from build123d import *

# Parameters (mm, degrees)
F0_W     = 118
F0_H     = 27.3
F0_W_2   = 114
F0_H_2   = 23.3
F1_DEPTH = 40
F2_W     = 4.2
F2_H     = 8.5
F3_DEPTH = 40
F4_W     = 27
F4_H     = 7.8
F5_DEPTH = 15
F6_W     = 118
F6_H     = 27.3
F7_DEPTH = 2


with BuildPart() as f1:
    # F0 (on Top) → F1 (new body)
    with BuildSketch(Plane.XY):
        with Locations((-1.233262, 0)):
            Rectangle(F0_W, F0_H)
        with Locations((-1.233262, 0)):
            Rectangle(F0_W_2, F0_H_2, mode=Mode.SUBTRACT)
    extrude(amount=F1_DEPTH)

    # F2 (on Top) → F3 (join)
    with BuildSketch(Plane.XY):
        with Locations((46.666738, 7.4)):
            Rectangle(F2_W, F2_H)
    extrude(amount=F3_DEPTH)

    # F4 (on Top) → F5 (join)
    with BuildSketch(Plane.XY):
        with Locations((35.266738, -7.75)):
            Rectangle(F4_W, F4_H)
    extrude(amount=F5_DEPTH)

    # F6 (on Top) → F7 (join)
    with BuildSketch(Plane.XY):
        with Locations((-1.233262, 0)):
            Rectangle(F6_W, F6_H)
    extrude(amount=-F7_DEPTH)


solid = f1.part
Read the model definition and answer for the solid it produces. Units are mm, in the model's axes. A direction names the side the tool comes from. Give positions to 0.01 mm unless a question says otherwise; leave off trailing zeros. Write each loop counter-clockwise with the first axis right and the second up, starting at its lowest first coordinate (ties: lowest second). Pieces come first, ordered by that corner, then holes. Notation, with made-up numbers: (-7, 46.5) - (48, 46.5) arc R23 ccw to (48, 68.5) - close; hole circle Ø6 at (50.5, 35). An arc over 180 degrees is marked (long way). Return JSON: item names as keys, results as strings.
Q1. Given P1, Ø8.5, axis at x = 38, y = -6, coming from the +Z side; P2, Ø1.5, axis at x = 43, y = 8, coming from the +Z side, each flat-ended and moving along its own axis, determine where each tip first touches the part or whether it passes through.
Reply:
{"P1": "z = 15", "P2": "z = 0"}
Q2. A cutting plane is placed at D-D, the plane x = 31. Determine the outline of the cut face in (y, z), and give its area (3 significant figures).
Reply:
{"outline": "(-13.65, -2) - (13.65, -2) - (13.65, 40) - (11.65, 40) - (11.65, 0) - (-3.85, 0) - (-3.85, 15) - (-11.65, 15) - (-11.65, 40) - (-13.65, 40) - close", "area": "332 mm²"}
Q3. For faces 4 (the face through (-8, 11.65, 20)), 5 (the face through (-2, 13.65, 19)), determine the directions among +Z, -Z, +X, -X, +Y, -Y from which every point of the face is accessible in a straight line to the end or side of a thin tool.
Reply:
{"face 4": "+Z", "face 5": "+Z, -Z, +X, -X, +Y"}
Q4. Consider line 1 along X through (y, z) = (-7, 9.5); line 2 along X through (y, z) = (4.75, 38); line 3 along Y through (x, z) = (31, 13). Determine where each line is inside the solid, lowest interval first. Write a range as [from, to].
Reply:
{"line 1": "[-60.23, -58.23], [21.77, 48.77], [55.77, 57.77]", "line 2": "[-60.23, -58.23], [44.57, 48.77], [55.77, 57.77]", "line 3": "[-13.65, -3.85], [11.65, 13.65]"}
Q5. A cutting plane is placed at C-C, the plane y = 8. Determine the outline of the cut face in (x, z).
Reply:
{"outline": "(-60.23, -2) - (57.77, -2) - (57.77, 40) - (55.77, 40) - (55.77, 0) - (48.77, 0) - (48.77, 40) - (44.57, 40) - (44.57, 0) - (-58.23, 0) - (-58.23, 40) - (-60.23, 40) - close"}
Q6. A cutting plane is placed at B-B, the plane x = -7.5. Determine the outline of the cut face in (y, z), and give its area (3 significant figures).
Reply:
{"outline": "(-13.65, -2) - (13.65, -2) - (13.65, 40) - (11.65, 40) - (11.65, 0) - (-11.65, 0) - (-11.65, 40) - (-13.65, 40) - close", "area": "215 mm²"}
Q7. A cutting plane is placed at A-A, the plane z = 4. Determine the outline of the cut face in (x, y).
Reply:
{"outline": "(-60.23, -13.65) - (57.77, -13.65) - (57.77, 13.65) - (-60.23, 13.65) - close; hole (-58.23, -11.65) - (21.77, -11.65) - (21.77, -3.85) - (48.77, -3.85) - (48.77, -11.65) - (55.77, -11.65) - (55.77, 11.65) - (48.77, 11.65) - (48.77, 3.15) - (44.57, 3.15) - (44.57, 11.65) - (-58.23, 11.65) - close"}
Q8. For a pull along X with two mould halves and no side action, classify faces 1 (the face through (47, 3.15, 20)), 2 (the face through (-60.233, 0, 19)), 3 (the face through (57.767, 0, 19)) as released by +X, released by -X, zero draft, split by the parting line, or undercut.
Reply:
{"face 1": "undercut", "face 2": "released by -X", "face 3": "released by +X"}
